```python
from build123d import *

# Parameters (mm, degrees)
F1_DEPTH = 63.5
F2_DEPTH = 25.4
F3_DEPTH = 7.9375
F0_W     = 25.4
F0_H     = 19.05
F4_DEPTH = 25.4
F6_R     = 6.35


with BuildPart() as f1:
    # F0 (on Front) → F1 (new body, symmetric)
    with BuildSketch(Plane.XZ):
        Polygon((41.275, -9.525), (41.275, 9.525), (22.225, 9.525), (-41.275, 9.525), (-41.275, -9.525), align=None)
    extrude(amount=F1_DEPTH, both=True)

    # F0 (on Front) → F2 (join, symmetric)
    with BuildSketch(Plane.XZ):
        with BuildLine():
            Line((22.225, 9.525), (41.275, 9.525))
            Line((41.275, 9.525), (41.275, 27.0002))
            ThreePointArc((41.275, 27.0002), (45.9246798487, 38.2255201513), (57.15, 42.8752))
            Line((57.15, 42.8752), (60.325, 42.8752))
            Line((60.325, 42.8752), (60.325, 61.9252))
            Line((60.325, 61.9252), (57.15, 61.9252))
            ThreePointArc((57.15, 61.9252), (32.4542956671, 51.6959043329), (22.225, 27.0002))
            Line((22.225, 27.0002), (22.225, 9.525))
        make_face()
    extrude(amount=F2_DEPTH, both=True)

    # F0 (on Front) → F3 (join, symmetric)
    with BuildSketch(Plane.XZ):
        with BuildLine():
            Line((-41.275, 9.525), (22.225, 9.525))
            Line((22.225, 9.525), (22.225, 27.0002))
            ThreePointArc((22.225, 27.0002), (32.4542956671, 51.6959043329), (57.15, 61.9252))
            add(Edge.make_bspline(
                [(-41.275, 9.525), (-41.1688275635, 34.6403568983), (17.4624975771, 62.293600291), (57.15, 61.9252)],
                knots=[0, 0, 0, 0, 111.5045361635, 111.5045361635, 111.5045361635, 111.5045361635], degree=3))
        make_face()
    extrude(amount=F3_DEPTH, both=True)

    # F0 (on Front) → F4 (join, symmetric)
    with BuildSketch(Plane.XZ):
        with Locations((73.025, 52.4002)):
            Rectangle(F0_W, F0_H)
    extrude(amount=F4_DEPTH, both=True)

    # F0 (on Front) → F5 (revolve)
    with BuildSketch(Plane.XZ):
        Polygon((85.725, 61.9252), (85.725, 42.8752), (85.725, 38.1), (111.125, 38.1), (111.125, 66.675), (85.725, 66.675), align=None)
    revolve(axis=Axis((85.725, 0, 52.3875), (0, 0, -1)))

    # F6
    f6_edges = [f1.edges().sort_by_distance(p)[0] for p in [
        (41.275, -63.5, 0),
        (-41.275, -63.5, 0),
        (41.275, 63.5, 0),
        (-41.275, 63.5, 0),
    ]]
    fillet(f6_edges, radius=F6_R)


solid = f1.part
```
The model under review builds one solid part; all positions refer to its coordinate system, in mm. A direction names the side the tool comes from. Round coordinates to 2 decimals unless told otherwise and drop trailing zeros. Loops run counter-clockwise (first coordinate to the right, second up) from the corner with the lowest first, then second, coordinate; pieces in that order, holes last. Notation, with made-up numbers: (41, 49) - (74, 49) arc R21 ccw to (74, 67) - close; hole circle Ø5 at (85.25, -25.5). An arc over 180 degrees is marked (long way). Use a Markdown table: item, result. Add a question column.
Q1. Add section A-A (z = -3). State the section outline as (x, y) points (3 decimals).
Q2. The part is to be moulded in two halves that separate along Z. For faces 6 (the face through (86, 0, 38.1)), 7 (the face through (32.73, 16.55, 51.97)), 8 (the face through (39.464, -61.59, 0.133)), say which applies: pulls with the +Z half, pulls with the -Z half, needs draft (parallel to the pull), parting line crosses it, or undercut.
Q3. Add section B-B (x = 66.5). State the section outline as (y, z) points (3 decimals), plus the area to 3 significant figures.
Q4. Machinability: for faces 1 (the face through (22.225, 17, 18)), 2 (the face through (46, 25.4, 42)), 3 (the face through (32.73, -16.79, 51.97)), 4 (the face through (46, -25.4, 42)), 5 (the face through (41.275, -1, 4)), which of the approach directions +Z, -Z, +X, -X, +Y, -Y give a long, thin tool a straight path to every point of the face, cutting with its end or side? Answer none if there is none.
Q5. For probe 1 along X at (y, z) = (-44.5, -2.5) (3 decimals); probe 2 along Z at (x, y) = (101, -13) (3 decimals); probe 3 along Y at (x, z) = (11, 39), list the stretches that pass through material, from the lowest coordinate up.
Q6. Insertion check: pin 1 Ø15.5 at (x, z) = (50.5, 45.5) entering from -Y; pin 2 Ø15.5 at (x, z) = (-6.5, 39) entering from -Y; pin 3 Ø8.5 at (x, y) = (65, -12.5) entering from -Z. Each pin has a flat end and moves straight along its axis. Give the tip position at first contact, or say it passes through.
Q7. Add section D-D (y = -28.5). State the section outline as (x, z) points (3 decimals), plus the area to 3 significant figures.
Q8. Add section C-C (y = -13.5). State the section outline as (x, z) points (3 decimals).
Worked answers:
| question | item | result |
|---|---|---|
| 1 | outline | (-41.275, -57.15) arc R6.35 ccw to (-34.925, -63.5) - (34.925, -63.5) arc R6.35 ccw to (41.275, -57.15) - (41.275, 57.15) arc R6.35 ccw to (34.925, 63.5) - (-34.925, 63.5) arc R6.35 ccw to (-41.275, 57.15) - close |
| 2 | face 6 | pulls with the -Z half |
| 2 | face 7 | pulls with the +Z half |
| 2 | face 8 | needs draft |
| 3 | outline | (-25.4, 42.875) - (-16.6, 42.875) - (-16.6, 38.1) - (16.6, 38.1) - (16.6, 42.875) - (25.4, 42.875) - (25.4, 61.925) - (16.6, 61.925) - (16.6, 66.675) - (-16.6, 66.675) - (-16.6, 61.925) - (-25.4, 61.925) - close |
| 3 | area | 1,280 mm² |
| 4 | face 1 | +Z, -X, +Y |
| 4 | face 2 | +Z, +X, -X, +Y |
| 4 | face 3 | +Z, -X, -Y |
| 4 | face 4 | +Z, +X, -X, -Y |
| 4 | face 5 | -Z, +X, +Y, -Y |
| 5 | probe 1 | -41.275 to 41.275 |
| 5 | probe 2 | 38.1 to 66.675 |
| 5 | probe 3 | -7.94 to 7.94 |
| 6 | pin 1 | y = -25.4 |
| 6 | pin 2 | y = -7.94 |
| 6 | pin 3 | z = 38.1 |
| 7 | outline | (-41.275, -9.525) - (41.275, -9.525) - (41.275, 9.525) - (-41.275, 9.525) - close |
| 7 | area | 1,570 mm² |
| 8 | outline | (-41.275, -9.525) - (41.275, -9.525) - (41.275, 27) arc R15.875 cw to (57.15, 42.875) - (64.21, 42.875) - (64.21, 38.1) - (107.24, 38.1) - (107.24, 66.675) - (64.21, 66.675) - (64.21, 61.925) - (57.15, 61.925) arc R34.925 ccw to (22.225, 27) - (22.225, 9.525) - (-41.275, 9.525) - close |
